Check sheet for the modelled part. Datum: model origin and axes. Units: mm. A direction names the side the tool comes from. Give positions to 0.01 mm unless a question says otherwise; leave off trailing zeros. Order: outer loops, then holes, each group sorted by start corner. A loop starts at its lowest first (then second) coordinate and runs counter-clockwise, first axis right, second up.
Item 1: Release check for a two-part mould opening along X. For faces 3 (the cylindrical face through (-3.86, 1.65, -5.04)), 4 (the flat face through (3, 6.35, -2)), 5 (the flat face through (0, 0, 0)) record: released by +X, released by -X, zero draft, split by the parting line, or undercut.
Item 2: Material ranges on line 1 along X through (y, z) = (3.25, 0) (3 decimals); line 2 along X through (y, z) = (0.75, -1); line 3 along Y through (x, z) = (1.5, -2), recorded low to high.
Item 3: Gauge pin test, flat ends, axial feed: P1, Ø6, axis at y = 1.5, z = 4, coming from the +X side; P2, Ø2, axis at x = 3, y = 4, coming from the +Z side; P3, Ø3, axis at x = -0.5, z = 0.5, coming from the +Y side. Record the tip position at first contact, or that the pin passes through.
Item 4: Access from +Z, -Z, +X, -X, +Y, -Y to the whole of each face (thin tool, end or side, straight path). Record for faces 1 (the cylindrical face through (-1.93, 3.22, -2.52)), 2 (the flat face through (0, -6.35, 0)).
Item 5: Sectioned sample at A-A on y = 0.75. Record the boundary of the cut face in (x, z) (3 decimals), and give its area (3 significant figures).
from build123d import *

# Parameters (mm, degrees)
SKETCH1_R           = 6.35
BOSS_EXTRUDE1_DEPTH = 6.35
SKETCH2_R           = 3.175
CUT_EXTRUDE1_DEPTH  = 6.35
FILLET1_R           = 3.175


with BuildPart() as part:
    # Sketch1 → Boss-Extrude1 (new, symmetric)
    with BuildSketch(Plane(origin=(0, 0, 0), x_dir=(1, 0, 0), z_dir=(0, 1, 0))):
        with Locations(Location((0, 0, 0), (0, 0, 270))):
            Circle(SKETCH1_R)
    extrude(amount=BOSS_EXTRUDE1_DEPTH, both=True)

    # Sketch2 → Cut-Extrude1 (cut)
    with BuildSketch(Plane(origin=(0, 6.35, 0), x_dir=(1, 0, 0), z_dir=(0, 1, 0))):
        with Locations(Location((0, 0, 0), (0, 0, 270))):
            Circle(SKETCH2_R)
    extrude(amount=-CUT_EXTRUDE1_DEPTH, mode=Mode.SUBTRACT)

    # Fillet1
    fillet1_edges = [part.edges().sort_by_distance(p)[0] for p in [
        (0, -6.35, -6.35),
    ]]
    fillet(fillet1_edges, radius=FILLET1_R)


solid = part.part
Report:
1. face 3: split by the parting line
1. face 4: zero draft
1. face 5: undercut
2. line 1: x = -6.35 to -3.175, 3.175 to 6.35
2. line 2: x = -6.27 to -3.01, 3.01 to 6.27
2. line 3: y = -6.35 to 0
3. P1: stops at x = 6.27
3. P2: stops at z = 6.03
3. P3: stops at y = 0
4. face 1: +Y
4. face 2: +Z, -Z, +X, -X, -Y
5. outline: circle Ø12.7 at (0, 0); hole circle Ø6.35 at (0, 0)
5. area: 95.0 mm2
